Design review of the part built by this model. Coordinates are the model's own, in mm. A direction names the side the tool comes from. Give positions to 0.01 mm unless a question says otherwise; leave off trailing zeros. Loops run counter-clockwise (first coordinate to the right, second up) from the corner with the lowest first, then second, coordinate; pieces in that order, holes last.
from build123d import *

# Parameters (mm, degrees)
F0_W     = 150
F0_H     = 90
F1_DEPTH = 30
F2_T     = -2.5
F3_R     = 10
F4_R     = 5


with BuildPart() as f1:
    # F0 (on Top) → F1 (new body)
    with BuildSketch(Plane.XY):
        Rectangle(F0_W, F0_H)
    extrude(amount=F1_DEPTH)

    # F2
    f2_openings = [f1.faces().sort_by_distance(p)[0] for p in [
        (0, 0, 30),
    ]]
    offset(amount=F2_T, openings=f2_openings)

    # F3
    f3_edges = [f1.edges().sort_by_distance(p)[0] for p in [
        (-75, 45, 15),
        (75, 45, 15),
        (75, -45, 15),
        (-75, -45, 15),
        (-72.5, 42.5, 16.25),
        (72.5, 42.5, 16.25),
        (72.5, -42.5, 16.25),
        (-72.5, -42.5, 16.25),
    ]]
    fillet(f3_edges, radius=F3_R)

    # F4
    f4_edges = [f1.edges().sort_by_distance(p)[0] for p in [
        (-75, 0, 0),
        (-72.071068, -42.071068, 0),
        (0, -45, 0),
        (72.071068, -42.071068, 0),
        (75, 0, 0),
        (72.071068, 42.071068, 0),
        (0, 45, 0),
        (-72.071068, 42.071068, 0),
    ]]
    fillet(f4_edges, radius=F4_R)


solid = f1.part
Q1. Wall thickness on line 1 (X direction, y = 24, z = 24.25); line 2 (Y direction, x = -24, z = 14); line 3 (Z direction, x = -3.5, y = 16): over which ranges is each line inside the solid? List them lowest first.
Results:
line 1: x = -75 to -72.5, 72.5 to 75
line 2: y = -45 to -42.5, 42.5 to 45
line 3: z = 0 to 2.5
Q2. Tool access review of faces 4 (the face through (-74, 0, 2)), 5 (the face through (-1, 42.5, 16)): name each direction out of +Z, -Z, +X, -X, +Y, -Y from which nothing blocks a thin tool from reaching the whole face with its end or side.
Results:
face 4: -Z, -X, +Y, -Y
face 5: +Z
Q3. Draft analysis for pull direction X (two halves, no side actions). For faces 1 (the face through (-75, 0, 17)), 2 (the face through (1, 44, 2)), 3 (the face through (-1, -42.5, 16)), state which applies: pulls with the +X half, pulls with the -X half, needs draft (parallel to the pull), parting line crosses it, or undercut.
Results:
face 1: pulls with the -X half
face 2: needs draft
face 3: undercut
Q4. Take a section at A-A (z = 22.75). Give the boundary of the cut face in (x, y).
Results:
outline: (-75, -35) arc R10 ccw to (-65, -45) - (65, -45) arc R10 ccw to (75, -35) - (75, 35) arc R10 ccw to (65, 45) - (-65, 45) arc R10 ccw to (-75, 35) - close; hole (-72.5, -32.5) arc R10 ccw to (-62.5, -42.5) - (62.5, -42.5) arc R10 ccw to (72.5, -32.5) - (72.5, 32.5) arc R10 ccw to (62.5, 42.5) - (-62.5, 42.5) arc R10 ccw to (-72.5, 32.5) - close
Q5. Take a section at B-B (y = 23). Give the boundary of the cut face in (x, z), plus the area to 3 significant figures.
Results:
outline: (-75, 5) arc R5 ccw to (-70, 0) - (70, 0) arc R5 ccw to (75, 5) - (75, 30) - (72.5, 30) - (72.5, 2.5) - (-72.5, 2.5) - (-72.5, 30) - (-75, 30) - close
area: 502 mm2
Q6. Take a section at C-C (x = -31.5). Give the boundary of the cut face in (y, z).
Results:
outline: (-45, 5) arc R5 ccw to (-40, 0) - (40, 0) arc R5 ccw to (45, 5) - (45, 30) - (42.5, 30) - (42.5, 2.5) - (-42.5, 2.5) - (-42.5, 30) - (-45, 30) - close
